Input: part model. Units: mm. Frame: model coordinates. A direction names the side the tool comes from. Round coordinates to 2 decimals unless told otherwise and drop trailing zeros. Loops run counter-clockwise (first coordinate to the right, second up) from the corner with the lowest first, then second, coordinate; pieces in that order, holes last. Notation, with made-up numbers: M -33.5,64 L -26.5,64 A29 cw -26.5,86 Z; hole C 50.5,-22.75 d4. An arc over 180 degrees is marked long. Return JSON: item names as keys, results as strings. Group by question number.
1) Contact query for flat-ended pins moving along their axis: P1, Ø0.5, axis at y = -2.5, z = 16.5, coming from the -X side; P2, Ø0.9, axis at x = 57.5, z = 16, coming from the +Y side; P3, Ø1.1, axis at x = 56, y = -2, coming from the +Z side. Output: stop coordinate, or through.
2) Section D-D (z = 16.25). Output: boundary loops of the cut face in (x, y), plus the area to 3 significant figures.
3) Section C-C (x = 57.8). Output: boundary loops of the cut face in (y, z), plus the area to 3 significant figures.
4) Access query for faces 1 (the face through (58, -0.65, 16)), 2 (the face through (56, -2, 14.8)), 3 (the face through (58, -2, 14.2)). Directions: +Z, -Z, +X, -X, +Y, -Y. A direction counts if a zero-diameter tool reaches every point of the face in a straight line with its end or side. Return the directions, or none.
5) Material intervals for line 1 (X direction, y = -0.75, z = 13); line 2 (Y direction, x = 57.55, z = 17); line 3 (Z direction, x = 59.45, y = -3.5), sorted ascending. Write a range as from..to.
6) Section B-B (z = 14.5). Output: boundary loops of the cut face in (x, y), plus the area to 3 significant figures.
7) Mould query, pull axis Y, two halves, no side actions, for faces 4 (the face through (56, -6.25, 14)), 5 (the face through (56, -2.9, 16)), 6 (the face through (56, -2, 10.2)). Classes: +Y half, -Y half, draft (parallel to the pull), parting line (faces both ways), or undercut.
8) Section A-A (y = -1.75). Output: boundary loops of the cut face in (x, z), plus the area to 3 significant figures.
from build123d import *

# Parameters (mm, degrees)
SKETCH047_W     = 3
SKETCH047_H     = 3.6
PAD020_DEPTH    = 3
SKETCH048_W     = 8.2
SKETCH048_H     = 7.6
PAD021_DEPTH    = 1
SKETCH053_W     = 1.6
SKETCH053_H     = 1
POCKET018_DEPTH = 3


with BuildPart() as part:
    # Sketch047 → Pad020 (new body)
    with BuildSketch(Plane.YZ.offset(56.6)):
        with Locations((-2.15, 16)):
            Rectangle(SKETCH047_W, SKETCH047_H)
    extrude(amount=PAD020_DEPTH)

    # Sketch048 (on Face5 of Pad020) → Pad021 (join)
    with BuildSketch(Plane(origin=(56.6, 0, 0), x_dir=(0, 1, 0), z_dir=(-1, 0, 0))):
        with Locations((-2.15, -14)):
            Rectangle(SKETCH048_W, SKETCH048_H)
    extrude(amount=PAD021_DEPTH)

    # Sketch053 (on Face6 of Pad021) → Pocket018 (cut)
    with BuildSketch(Plane(origin=(0, 0, 17.8), x_dir=(0, -1, 0), z_dir=(0, 0, 1))):
        with Locations((2.1, 56.1)):
            Rectangle(SKETCH053_W, SKETCH053_H)
    extrude(amount=-POCKET018_DEPTH, mode=Mode.SUBTRACT)


solid = part.part
Returned:
{
 "1": {"P1": "stops at x = 56.6", "P2": "stops at y = -0.65", "P3": "stops at z = 14.8"},
 "2": {"outline": "M 55.6,-6.25 L 56.6,-6.25 L 56.6,-3.65 L 59.6,-3.65 L 59.6,-0.65 L 56.6,-0.65 L 56.6,1.95 L 55.6,1.95 L 55.6,-1.3 L 56.6,-1.3 L 56.6,-2.9 L 55.6,-2.9 Z", "area": "15.6 mm^2"},
 "3": {"outline": "M -3.65,14.2 L -0.65,14.2 L -0.65,17.8 L -3.65,17.8 Z", "area": "10.8 mm^2"},
 "4": {"face 1": "+Z, -Z, +X, +Y", "face 2": "+Z, -X", "face 3": "-Z, +X, +Y, -Y"},
 "5": {"line 1": "x = 55.6..56.6", "line 2": "y = -3.65..-0.65", "line 3": "z = 14.2..17.8"},
 "6": {"outline": "M 55.6,-6.25 L 56.6,-6.25 L 56.6,-3.65 L 59.6,-3.65 L 59.6,-0.65 L 56.6,-0.65 L 56.6,1.95 L 55.6,1.95 Z", "area": "17.2 mm^2"},
 "7": {"face 4": "-Y half", "face 5": "undercut", "face 6": "draft"},
 "8": {"outline": "M 55.6,10.2 L 56.6,10.2 L 56.6,14.2 L 59.6,14.2 L 59.6,17.8 L 56.6,17.8 L 56.6,14.8 L 55.6,14.8 Z", "area": "15.4 mm^2"}
}
